Here's how the part is built. I have some questions about the finished solid (model axes, mm). Face numbers are marked on the shaded views. A direction names the side the tool comes from. Round coordinates to 2 decimals unless told otherwise and drop trailing zeros. Loops run counter-clockwise (first coordinate to the right, second up) from the corner with the lowest first, then second, coordinate; pieces in that order, holes last. Notation, with made-up numbers: M 71,49.25 L 114,49.25 A19 ccw 114,79.25 Z; hole C 57.5,1.25 d5. An arc over 180 degrees is marked long. Use a Markdown table: item, result.
```python
from build123d import *

# Parameters (mm, degrees)
ESQUISSE1_W             = 20
ESQUISSE1_H             = 17
ESQUISSE1_R             = 2.1
BOSS_EXTRU_1_DEPTH      = 5
ESQUISSE2_W             = 18
ESQUISSE2_H             = 3
BOSS_EXTRU_3_DEPTH      = 24
ESQUISSE5_W             = 6.5
ESQUISSE5_H             = 17
ENL_V_MAT_EXTRU_3_DEPTH = 18
ESQUISSE10_W            = 7
ESQUISSE10_H            = 3
BOSS_EXTRU_6_DEPTH      = 10
ESQUISSE11_W            = 5.5
ESQUISSE11_H            = 2.5
ESQUISSE11_W_2          = 7
ESQUISSE11_H_2          = 0.5
BOSS_EXTRU_7_DEPTH      = 17
ESQUISSE12_W            = 18
ESQUISSE12_H            = 2.5
BOSS_EXTRU_8_DEPTH      = 24
CONG_3_R                = 9
ESQUISSE20_R            = 2.25
ENL_V_MAT_EXTRU_7_DEPTH = 18
ESQUISSE22_W            = 7
ESQUISSE22_H            = 5
BOSS_EXTRU_9_DEPTH      = 23
ESQUISSE27_W            = 5.5
ESQUISSE27_H            = 5
ESQUISSE27_W_2          = 7
BOSS_EXTRU_10_DEPTH     = 24
CONG_4_R                = 9
ESQUISSE28_R            = 2.75
ENL_V_MAT_EXTRU_8_DEPTH = 44
CONG_5_R                = 1
CONG_6_R                = 5.5


with BuildPart() as part:
    # Esquisse1 → Boss.-Extru.1 (new body)
    with BuildSketch(Plane.XY):
        with Locations((10, 8.5)):
            Rectangle(ESQUISSE1_W, ESQUISSE1_H)
        with Locations((10, 5)):
            Circle(ESQUISSE1_R, mode=Mode.SUBTRACT)
        with Locations((10, 12)):
            Circle(ESQUISSE1_R, mode=Mode.SUBTRACT)
    extrude(amount=BOSS_EXTRU_1_DEPTH)

    # Esquisse5 → Enlèv. mat.-Extru.3 (cut)
    with BuildSketch(Plane.XY.offset(5)):
        with Locations((16.75, 8.5)):
            Rectangle(ESQUISSE5_W, ESQUISSE5_H)
        with Locations((3.25, 8.5)):
            Rectangle(ESQUISSE5_W, ESQUISSE5_H)
    extrude(amount=-ENL_V_MAT_EXTRU_3_DEPTH, mode=Mode.SUBTRACT)



with BuildPart() as body_2:
    # Esquisse2 → Boss.-Extru.3 (new body)
    with BuildSketch(Plane.XZ):
        with Locations((10, -3.5)):
            Rectangle(ESQUISSE2_W, ESQUISSE2_H)
    extrude(amount=BOSS_EXTRU_3_DEPTH)


with BuildPart() as part_1:
    add(part.part)

    add(body_2.part)  # Boss.-Extru.6 merges body 2
    # Esquisse10 → Boss.-Extru.6 (add)
    with BuildSketch(Plane.XY.offset(5)):
        with Locations((10, -1.5)):
            Rectangle(ESQUISSE10_W, ESQUISSE10_H)
    extrude(amount=-BOSS_EXTRU_6_DEPTH)

    # Esquisse11 → Boss.-Extru.7 (add)
    with BuildSketch(Plane(origin=(0, 0, 0), x_dir=(1, 0, 0), z_dir=(0, 1, 0))):
        with Locations((3.75, 6.25)):
            Rectangle(ESQUISSE11_W, ESQUISSE11_H)
        with Locations((10, 6.25)):
            Rectangle(ESQUISSE11_W_2, ESQUISSE11_H)
        with Locations((16.25, 6.25)):
            Rectangle(ESQUISSE11_W, ESQUISSE11_H)
        with Locations((3.75, 4.75)):
            Rectangle(ESQUISSE11_W, ESQUISSE11_H_2)
        with Locations((10, 4.75)):
            Rectangle(ESQUISSE11_W_2, ESQUISSE11_H_2)
        with Locations((16.25, 4.75)):
            Rectangle(ESQUISSE11_W, ESQUISSE11_H_2)
    extrude(amount=BOSS_EXTRU_7_DEPTH)

    # Esquisse12 → Boss.-Extru.8 (add)
    with BuildSketch(Plane.XZ):
        with Locations((10, -6.25)):
            Rectangle(ESQUISSE12_W, ESQUISSE12_H)
    extrude(amount=BOSS_EXTRU_8_DEPTH)

    # Congé3
    cong_3_edges = [part_1.edges().sort_by_distance(p)[0] for p in [
        (19, -24, -4.75),
        (1, -24, -4.75),
    ]]
    fillet(cong_3_edges, radius=CONG_3_R - 0.0001)  # a hair under: the kernel refuses the full size

    # Esquisse20 → Enlèv. mat.-Extru.7 (cut)
    with BuildSketch(Plane.XY.offset(5)):
        with Locations((10, 5)):
            Circle(ESQUISSE20_R)
        with Locations((10, 12)):
            Circle(ESQUISSE20_R)
    extrude(amount=-ENL_V_MAT_EXTRU_7_DEPTH, mode=Mode.SUBTRACT)

    # Esquisse22 → Boss.-Extru.9 (add)
    with BuildSketch(Plane.XY.offset(-2)):
        with Locations((10, -2.5)):
            Rectangle(ESQUISSE22_W, ESQUISSE22_H)
    extrude(amount=BOSS_EXTRU_9_DEPTH)

    # Esquisse27 → Boss.-Extru.10 (add)
    with BuildSketch(Plane(origin=(0, 0, 0), x_dir=(1, 0, 0), z_dir=(0, 1, 0))):
        with Locations((3.75, -18.5)):
            Rectangle(ESQUISSE27_W, ESQUISSE27_H)
        with Locations((16.25, -18.5)):
            Rectangle(ESQUISSE27_W, ESQUISSE27_H)
        with Locations((10, -18.5)):
            Rectangle(ESQUISSE27_W_2, ESQUISSE27_H)
    extrude(amount=-BOSS_EXTRU_10_DEPTH)

    # Congé4
    cong_4_edges = [part_1.edges().sort_by_distance(p)[0] for p in [
        (1, -24, 18.5),
        (19, -24, 18.5),
    ]]
    fillet(cong_4_edges, radius=CONG_4_R - 0.0001)  # a hair under: the kernel refuses the full size

    # Esquisse28 → Enlèv. mat.-Extru.8 (cut)
    with BuildSketch(Plane.XY.offset(21)):
        with Locations((10, -15)):
            Circle(ESQUISSE28_R)
    extrude(amount=-ENL_V_MAT_EXTRU_8_DEPTH, mode=Mode.SUBTRACT)

    # Congé5
    cong_5_edges = [part_1.edges().sort_by_distance(p)[0] for p in [
        (10, 0, 5),
        (10, -5, -2),
        (10, -5, 16),
        (6.5, -2.5, 16),
        (13.5, -2.5, 16),
        (6.5, -2.5, -2),
        (13.5, -2.5, -2),
    ]]
    fillet(cong_5_edges, radius=CONG_5_R)

    # Congé6
    cong_6_edges = [part_1.edges().sort_by_distance(p)[0] for p in [
        (1, 0, 18.5),
        (19, 0, 18.5),
    ]]
    fillet(cong_6_edges, radius=CONG_6_R - 0.0001)  # a hair under: the kernel refuses the full size


solid = part_1.part
```
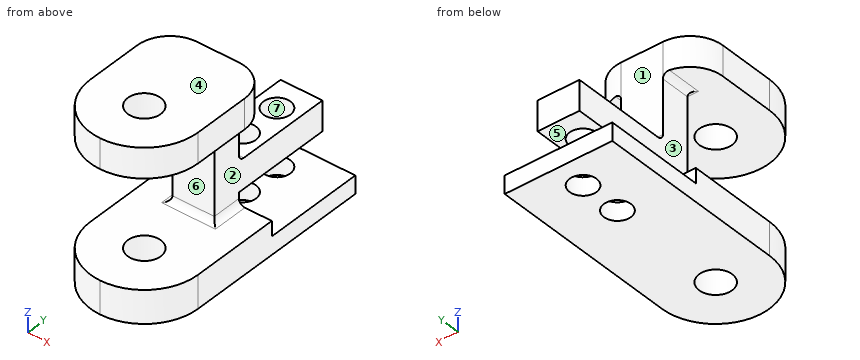
Q1. Imagine slicing it at D-D, the plane z = 14.25. Please give me the cut outline in (x, y), then the cut area to 3 significant figures.
Return value:
| item | result |
|---|---|
| outline | M 6.5,-5 L 13.5,-5 L 13.5,0 L 6.5,0 Z |
| area | 35.0 mm^2 |
Q2. For the marked faces 1, 2 and 3, which set-ups out of +Z, -Z, +X, -X, +Y, -Y let a thin tool reach every point of the face, with its end or its side?
Return value:
| item | result |
|---|---|
| face 1 | +Z, +X, -X, +Y |
| face 2 | +X, +Y, -Y |
| face 3 | -X, +Y, -Y |
Q3. Will these pins go through, and if not, where does the flat tip stop? P1, Ø12, axis at y = -5, z = 9, coming from the +X side; P2, Ø3.5, axis at x = 9, z = 7.5, coming from the -Y side; P3, Ø2.5, axis at x = 10, y = 5, coming from the +Z side; P4, Ø8.5, axis at x = 10.5, y = 9, coming from the +Z side.
Return value:
| item | result |
|---|---|
| P1 | stops at x = 13.5 |
| P2 | stops at y = -5 |
| P3 | passes through |
| P4 | stops at z = 5 |
Q4. Imagine slicing it at C-C, the plane x = 16. Please give me the cut outline in (y, z).
Return value:
| item | result |
|---|---|
| outline | M -21.71,-7.5 L 17,-7.5 L 17,-4.5 L 0,-4.5 L 0,-2 L -21.71,-2 Z; M -21.71,16 L -0.6,16 L -0.6,21 L -21.71,21 Z |
Q5. We'd pull the mould along Z, two halves only. Please class the marked faces 4, 5, 6 and 7: pulls with the +Z half, pulls with the -Z half, needs draft (parallel to the pull), parting line crosses it, or undercut.
Return value:
| item | result |
|---|---|
| face 4 | pulls with the +Z half |
| face 5 | undercut |
| face 6 | undercut |
| face 7 | needs draft |
Q6. Imagine slicing it at B-B, the plane y = 5. Please give me the cut outline in (x, z), then the cut area to 3 significant figures.
Return value:
| item | result |
|---|---|
| outline | M 1,-7.5 L 7.75,-7.5 L 7.75,-4.5 L 1,-4.5 Z; M 6.5,0 L 7.75,0 L 7.75,5 L 6.5,5 Z; M 12.25,-7.5 L 19,-7.5 L 19,-4.5 L 12.25,-4.5 Z; M 12.25,0 L 13.5,0 L 13.5,5 L 12.25,5 Z |
| area | 53.0 mm^2 |
Q7. Imagine slicing it at A-A, the plane y = -8. Please give me the cut outline in (x, z).
Return value:
| item | result |
|---|---|
| outline | M 1,-7.5 L 19,-7.5 L 19,-2 L 1,-2 Z; M 1,16 L 19,16 L 19,21 L 1,21 Z |
Q8. I need wall thicknesses on line 1 (Y direction, x = 10, z = 1.25); line 2 (Y direction, x = 10, z = -5.45); line 3 (Y direction, x = 10, z = 19.85). Which ranges of each line are inside material? Lowest first, please. Write a range as from..to.
Return value:
| item | result |
|---|---|
| line 1 | y = -5..2.75, 7.25..9.75, 14.25..17 |
| line 2 | y = -24..-17.75, -12.25..2.75, 7.25..9.75, 14.25..17 |
| line 3 | y = -24..-17.75, -12.25..0 |
